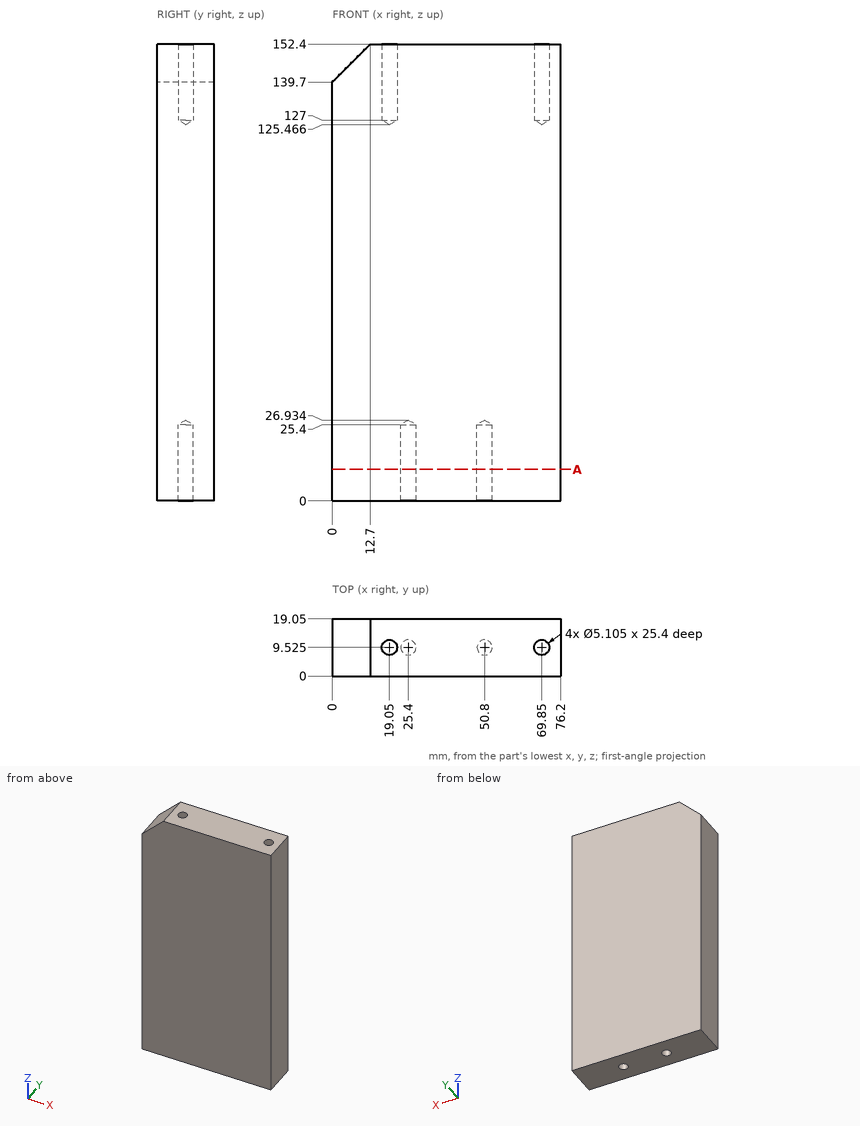
Design review of the part shown in the three views and the two pictorial views. Dimensions are in mm from the part's minimum x, y and z. Give positions to 0.01 mm unless a question says otherwise; leave off trailing zeros. Answer in a Markdown table with one row per item. Add a question column.
(1) For pin 1 (4.5 mm diameter, centred on x = 69.85, y = 9.525, fed in from +Z), flat-tipped, find the tip position at first contact; note if it passes through.
(2) Wall thickness on probe 1 along Y at (x, z) = (69.85, 138); probe 2 along X at (y, z) = (8.25, 130); probe 3 along Z at (x, y) = (69.5, 7.5): over which ranges is each line inside the solid? List them lowest first. Write a range as [from, to].
(3) Consider section A-A on z = 10.5. Give the number of separate pieces and of enclosed holes in the cut face, and give its area (3 significant figures).
Evaluation:
| question | item | result |
|---|---|---|
| 1 | pin 1 | stops at z = 126.82 |
| 2 | probe 1 | y = [0, 6.97], [12.08, 19.05] |
| 2 | probe 2 | x = [0, 16.84], [21.26, 67.64], [72.06, 76.2] |
| 2 | probe 3 | z = [0, 126.7] |
| 3 | separate pieces | 1 |
| 3 | enclosed holes | 2 |
| 3 | area | 1,410 mm^2 |
